Part model, mm, in its own coordinate system. Face numbers are marked on the shaded views. A direction names the side the tool comes from. Give positions to 0.01 mm unless a question says otherwise; leave off trailing zeros. Write each loop counter-clockwise with the first axis right and the second up, starting at its lowest first coordinate (ties: lowest second). Pieces come first, ordered by that corner, then holes. Notation, with made-up numbers: M -1.5,25 L 42.5,25 A31 cw 42.5,58 Z; hole C 81,64 d4. An arc over 180 degrees is marked long. Use a Markdown table: item, result.
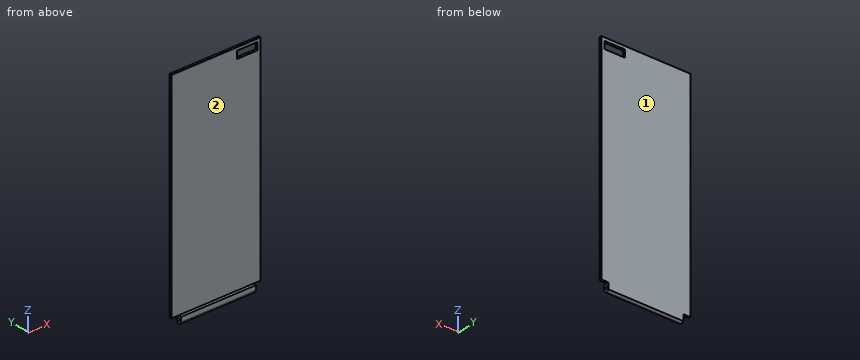
```python
from build123d import *

# Parameters (mm, degrees)
SKETCH1_W           = 30
SKETCH1_H           = 70
BOSS_EXTRUDE1_DEPTH = 1
SKETCH5_W           = 30
SKETCH5_H           = 1
BOSS_EXTRUDE3_DEPTH = 5
SKETCH6_W           = 7
SKETCH6_H           = 2.5
CUT_EXTRUDE3_DEPTH  = 1
SKETCH2_W           = 30
SKETCH2_H           = 2.5
BOSS_EXTRUDE4_DEPTH = 1
CUT_EXTRUDE4_START  = -30
SKETCH7_R           = 0.5
CUT_EXTRUDE4_DEPTH  = 30
FILLET1_R           = 1
SKETCH9_W           = 3
SKETCH9_H           = 2
CUT_EXTRUDE5_DEPTH  = 2.5
SKETCH10_W          = 3
SKETCH10_H          = 2
CUT_EXTRUDE6_DEPTH  = 2.5
SKETCH11_W          = 33.967551934
SKETCH11_H          = 76.426629991
CUT_EXTRUDE7_DEPTH  = 0.2


with BuildPart() as part:
    # Sketch1 → Boss-Extrude1 (new body)
    with BuildSketch(Plane(origin=(0, 0, 0), x_dir=(1, 0, 0), z_dir=(0, 1, 0))):
        Rectangle(SKETCH1_W, SKETCH1_H)
    extrude(amount=BOSS_EXTRUDE1_DEPTH)

    # Sketch5 → Boss-Extrude3 (add)
    with BuildSketch(Plane.XY.offset(35)):
        with Locations((0, 0.5)):
            Rectangle(SKETCH5_W, SKETCH5_H)
    extrude(amount=BOSS_EXTRUDE3_DEPTH)

    # Sketch6 → Cut-Extrude3 (cut)
    with BuildSketch(Plane(origin=(0, 1, 0), x_dir=(1, 0, 0), z_dir=(0, 1, 0))):
        with Locations((10.5, -37.75)):
            Rectangle(SKETCH6_W, SKETCH6_H)
    extrude(amount=-CUT_EXTRUDE3_DEPTH, mode=Mode.SUBTRACT)

    # Sketch2 → Boss-Extrude4 (add)
    with BuildSketch(Plane(origin=(0, 0, 0), x_dir=(1, 0, 0), z_dir=(0, 1, 0))):
        with Locations((0, 33.75)):
            Rectangle(SKETCH2_W, SKETCH2_H)
    extrude(amount=-BOSS_EXTRUDE4_DEPTH)

    # Sketch7 → Cut-Extrude4 (cut)
    with BuildSketch(Plane.ZY.offset(15).offset(CUT_EXTRUDE4_START)):
        with Locations((-33.75, 0)):
            Circle(SKETCH7_R)
    extrude(amount=CUT_EXTRUDE4_DEPTH, mode=Mode.SUBTRACT)

    # Fillet1
    fillet1_edges = [part.edges().sort_by_distance(p)[0] for p in [
        (0, -1, -35),
        (0, 1, -35),
    ]]
    fillet(fillet1_edges, radius=FILLET1_R - 0.0001)  # a hair under: the kernel refuses the full size

    # Sketch9 → Cut-Extrude5 (cut)
    with BuildSketch(Plane.ZY.offset(15)):
        with Locations((-34, 0)):
            Rectangle(SKETCH9_W, SKETCH9_H)
    extrude(amount=-CUT_EXTRUDE5_DEPTH, mode=Mode.SUBTRACT)

    # Sketch10 → Cut-Extrude6 (cut)
    with BuildSketch(Plane(origin=(15, 0, 0), x_dir=(0, 0, -1), z_dir=(1, 0, 0))):
        with Locations((34, 0)):
            Rectangle(SKETCH10_W, SKETCH10_H)
    extrude(amount=-CUT_EXTRUDE6_DEPTH, mode=Mode.SUBTRACT)

    # Sketch11 → Cut-Extrude7 (cut)
    with BuildSketch(Plane(origin=(0, 1, 0), x_dir=(1, 0, 0), z_dir=(0, 1, 0))):
        with Locations((-1.983775967, -1.786685004)):
            Rectangle(SKETCH11_W, SKETCH11_H)
    extrude(amount=-CUT_EXTRUDE7_DEPTH, mode=Mode.SUBTRACT)


solid = part.part
```
1. Cut at A-A, the plane x = 8.25. State how many separate pieces and enclosed holes the cut face has, then the cut area to 3 significant figures.
Findings below:
| item | result |
|---|---|
| separate pieces | 2 |
| enclosed holes | 1 |
| area | 59.4 mm2 |
2. Cut at C-C, the plane z = -6.5. Give the cut face in (x, y), then the cut area to 3 significant figures.
Findings below:
| item | result |
|---|---|
| outline | M -15,0 L 15,0 L 15,0.8 L -15,0.8 Z |
| area | 24.0 mm2 |
3. Drop flat-ended pins along their axis: P1, Ø4, axis at x = -6.5, z = -15, coming from the -Y side; P2, Ø0.9, axis at y = 0, z = -33.5, coming from the +X side. Give the stop position or say it passes through.
Findings below:
| item | result |
|---|---|
| P1 | y = 0 |
| P2 | x = 12.5 |
4. Tool access for the marked faces 1 and 2: list every direction of +Z, -Z, +X, -X, +Y, -Y with a clear straight run to the whole face (end or side of a thin tool).
Findings below:
| item | result |
|---|---|
| face 1 | +Z, -Z, +X, -X, +Y |
| face 2 | +Z, +X, -X, -Y |
5. Drill centre lines: L1, parallel to Y at x = -1.75, z = -33.75; L2, parallel to Z at x = 12.75, y = 0.45; L3, parallel to Z at x = 3.5, y = 0.1 (3 decimals). Where is each one in solid material? Low to high.
Findings below:
| item | result |
|---|---|
| L1 | -1 to -0.5, 0.5 to 0.8 |
| L2 | -32.5 to 36.5, 39 to 40 |
| L3 | -34.995 to -34.24, -33.26 to 40 |
